from build123d import *

# Parameters (mm, degrees)
EXTRUDE_LID_MAIN_DEPTH = 0.75
EXTRUDE_THIN2_DEPTH    = 0.75
UPPER_17_W             = 5
UPPER_17_H             = 1
UPPER_17_W_2           = 1
UPPER_17_H_2           = 2
LID_ANCHOR_FRONT_DEPTH = 4.5
TAP_LATERAL_LID_D      = 0.75
TAP_FRONT_LID_D        = 0.75
CUT_EXTRUDE1_REACH     = 16.029
HS_HOLDER_LID_DEPTH    = 7.5
M2_5_TAPPED_HOLE2_D    = 2.05


with BuildPart() as part:
    # upper<13> → extrude_lid_main (new body)
    with BuildSketch(Plane(origin=(0, -8, 0), x_dir=(1, 0, 0), z_dir=(0, 1, 0))):
        with BuildLine():
            Line((-6.250353693, -9.5), (6.250353693, -9.5))
            ThreePointArc((6.250353693, -9.5), (7.665029031, -8.913751636), (8.250353267, -7.498693688))
            ThreePointArc((8.250353267, -7.498693688), (8.248836384, -3.124346898), (8.25, 1.25))
            Line((8.25, 1.25), (8.25, 9.2))
            ThreePointArc((8.25, 9.2), (8.162132034, 9.412132034), (7.95, 9.5))
            Line((7.95, 9.5), (0.865, 9.5))
            Line((0.865, 9.5), (0.865, 4.5))
            Line((0.865, 4.5), (-3.935, 4.5))
            Line((-3.935, 4.5), (-3.935, 9.5))
            Line((-3.935, 9.5), (-7.95, 9.5))
            ThreePointArc((-7.95, 9.5), (-8.162132034, 9.412132034), (-8.25, 9.2))
            Line((-8.25, 9.2), (-8.25, 1.25))
            ThreePointArc((-8.25, 1.25), (-8.199296345, -3.106194095), (-8.25, -7.462388189))
            ThreePointArc((-8.25, -7.462388189), (-7.677803101, -8.900852665), (-6.250353693, -9.5))
        make_face()
    extrude(amount=EXTRUDE_LID_MAIN_DEPTH)



with BuildPart() as body_2:
    # upper<16> → Extrude-Thin2 (new body)
    with BuildSketch(Plane(origin=(0, -8, 0), x_dir=(1, 0, 0), z_dir=(0, 1, 0))):
        with BuildLine():
            Line((-8.75, 1.244176388), (-8.75, 9.2))
            ThreePointArc((-8.75, 9.2), (-8.515685425, 9.765685425), (-7.95, 10))
            Line((-7.95, 10), (7.95, 10))
            ThreePointArc((7.95, 10), (8.515685425, 9.765685425), (8.75, 9.2))
            Line((8.75, 9.2), (8.75, 1.249856897))
            ThreePointArc((8.75, 1.249856897), (8.748836381, -3.12425516), (8.75035316, -7.49836711))
            ThreePointArc((8.75035316, -7.49836711), (8.018697866, -9.267189545), (6.250353693, -10))
            Line((6.250353693, -10), (-6.250353693, -10))
            ThreePointArc((-6.250353693, -10), (-8.035078913, -9.250644422), (-8.749889093, -7.451804713))
            ThreePointArc((-8.749889093, -7.451804713), (-8.69929636, -3.103813517), (-8.75, 1.244176388))
        make_face()
        with BuildLine():
            Line((-8.25, 1.25), (-8.25, 9.2))
            ThreePointArc((-8.25, 9.2), (-8.162132034, 9.412132034), (-7.95, 9.5))
            Line((-7.95, 9.5), (7.95, 9.5))
            ThreePointArc((7.95, 9.5), (8.162132034, 9.412132034), (8.25, 9.2))
            Line((8.25, 9.2), (8.25, 1.25))
            ThreePointArc((8.25, 1.25), (8.248836384, -3.124346898), (8.250353267, -7.498693688))
            ThreePointArc((8.250353267, -7.498693688), (7.665029031, -8.913751636), (6.250353693, -9.5))
            Line((6.250353693, -9.5), (-6.250353693, -9.5))
            ThreePointArc((-6.250353693, -9.5), (-7.677803101, -8.900852665), (-8.25, -7.462388189))
            ThreePointArc((-8.25, -7.462388189), (-8.199296345, -3.106194095), (-8.25, 1.25))
        make_face(mode=Mode.SUBTRACT)
    extrude(amount=EXTRUDE_THIN2_DEPTH)


with BuildPart() as part_1:
    add(part.part)

    add(body_2.part)  # lid_anchor_front merges body 2
    # upper<17> → lid_anchor_front (add)
    with BuildSketch(Plane(origin=(0, -8, 0), x_dir=(1, 0, 0), z_dir=(0, 1, 0))):
        with Locations((0, -8.99)):
            Rectangle(UPPER_17_W, UPPER_17_H)
        with Locations((-7.74, 2.25)):
            Rectangle(UPPER_17_W_2, UPPER_17_H_2)
    lid_anchor_front = extrude(amount=-LID_ANCHOR_FRONT_DEPTH)

    # tap_lateral_lid (through all)
    with Locations(Plane.ZY.offset(8.24)):
        with Locations((-2.25, -11)):
            tap_lateral_lid = Hole(TAP_LATERAL_LID_D / 2)

    # Mirror3: lid_anchor_front, tap_lateral_lid across plane
    add(lid_anchor_front.mirror(Plane(origin=(0, 0, 0), x_dir=(0, 0, 1), z_dir=(1, 0, 0))))
    add(tap_lateral_lid.mirror(Plane(origin=(0, 0, 0), x_dir=(0, 0, 1), z_dir=(1, 0, 0))), mode=Mode.SUBTRACT)

    # tap_front_lid (through all)
    with Locations(Plane.XY.offset(9.49)):
        with Locations((0, -9)):
            Hole(TAP_FRONT_LID_D / 2)

    # upper<18> → Cut-Extrude1 (cut, up to next)
    with BuildSketch(Plane(origin=(0, -8, 0), x_dir=(1, 0, 0), z_dir=(0, 1, 0)), mode=Mode.PRIVATE) as cut_extrude1_sk1:
        with BuildLine():
            ThreePointArc((-2.5, 9.5), (-1.767766953, 11.267766953), (0, 12))
            Line((0, 12), (-1.556624327, 12))
            Line((-1.556624327, 12), (-3, 9.5))
            Line((-3, 9.5), (-2.5, 9.5))
        make_face()
    cut_extrude1_tool1 = extrude(cut_extrude1_sk1.sketch, amount=CUT_EXTRUDE1_REACH, mode=Mode.PRIVATE) & part_1.part
    # upper<18> → Cut-Extrude1 (cut, up to next)
    with BuildSketch(Plane(origin=(0, -8, 0), x_dir=(1, 0, 0), z_dir=(0, 1, 0)), mode=Mode.PRIVATE) as cut_extrude1_sk2:
        with BuildLine():
            Line((2.5, 9.5), (3, 9.5))
            Line((3, 9.5), (1.556624327, 12))
            Line((1.556624327, 12), (0, 12))
            ThreePointArc((0, 12), (1.767766953, 11.267766953), (2.5, 9.5))
        make_face()
    cut_extrude1_tool2 = extrude(cut_extrude1_sk2.sketch, amount=CUT_EXTRUDE1_REACH, mode=Mode.PRIVATE) & part_1.part
    # upper<18> → Cut-Extrude1 (cut, up to next)
    with BuildSketch(Plane(origin=(0, -8, 0), x_dir=(1, 0, 0), z_dir=(0, 1, 0)), mode=Mode.PRIVATE) as cut_extrude1_sk3:
        with BuildLine():
            Line((1.25, 9.5), (2.5, 9.5))
            ThreePointArc((2.5, 9.5), (1.767766953, 11.267766953), (0, 12))
            ThreePointArc((0, 12), (-1.767766953, 11.267766953), (-2.5, 9.5))
            Line((-2.5, 9.5), (-1.25, 9.5))
            Line((-1.25, 9.5), (0.865, 9.5))
            Line((0.865, 9.5), (1.25, 9.5))
        make_face()
    cut_extrude1_tool3 = extrude(cut_extrude1_sk3.sketch, amount=CUT_EXTRUDE1_REACH, mode=Mode.PRIVATE) & part_1.part
    # upper<18> → Cut-Extrude1 (cut, up to next)
    with BuildSketch(Plane(origin=(0, -8, 0), x_dir=(1, 0, 0), z_dir=(0, 1, 0)), mode=Mode.PRIVATE) as cut_extrude1_sk4:
        Polygon((1.556624327, 12), (3, 9.5), (3, 12), align=None)
    cut_extrude1_tool4 = extrude(cut_extrude1_sk4.sketch, amount=CUT_EXTRUDE1_REACH, mode=Mode.PRIVATE) & part_1.part
    # upper<18> → Cut-Extrude1 (cut, up to next)
    with BuildSketch(Plane(origin=(0, -8, 0), x_dir=(1, 0, 0), z_dir=(0, 1, 0)), mode=Mode.PRIVATE) as cut_extrude1_sk5:
        Polygon((-3, 9.5), (-1.556624327, 12), (-3.025026025, 12), (-3.025026025, 9.5), align=None)
    cut_extrude1_tool5 = extrude(cut_extrude1_sk5.sketch, amount=CUT_EXTRUDE1_REACH, mode=Mode.PRIVATE) & part_1.part
    add(cut_extrude1_tool1.solids().sort_by_distance((-2.75, -8, -9.539051))[0], mode=Mode.SUBTRACT)
    add(cut_extrude1_tool2.solids().sort_by_distance((2.244493, -8, -10.730474))[0], mode=Mode.SUBTRACT)
    add(cut_extrude1_tool3.solids().sort_by_distance((0, -8, -10.561033))[0], mode=Mode.SUBTRACT)
    add(cut_extrude1_tool4.solids().sort_by_distance((2.518875, -8, -11.166667))[0], mode=Mode.SUBTRACT)
    add(cut_extrude1_tool5.solids().sort_by_distance((-2.535419, -8, -11.152702))[0], mode=Mode.SUBTRACT)

    # upper<25> → hs-holder-lid (add)
    with BuildSketch(Plane(origin=(0, -8, 0), x_dir=(1, 0, 0), z_dir=(0, 1, 0))):
        Polygon((-8.25, 4.5), (-8.25, 3.5), (-2.25, 3.5), (-2.25, 4.5), (-3.935, 4.5), (-4.75, 4.5), align=None)
    hs_holder_lid = extrude(amount=-HS_HOLDER_LID_DEPTH)

    # M2.5 Tapped Hole2 (through all)
    with Locations(Plane(origin=(0, 0, -4.5), x_dir=(-1, 0, 0), z_dir=(0, 0, -1))):
        with Locations((4.25, -10.9)):
            m2_5_tapped_hole2 = Hole(M2_5_TAPPED_HOLE2_D / 2)

    # Mirror6: hs-holder-lid across plane
    add(hs_holder_lid.mirror(Plane(origin=(0, 0, 0), x_dir=(0, 0, 1), z_dir=(1, 0, 0))))

    # Mirror7: M2.5 Tapped Hole2 across plane
    add(m2_5_tapped_hole2.mirror(Plane(origin=(0, 0, 0), x_dir=(0, 0, 1), z_dir=(1, 0, 0))), mode=Mode.SUBTRACT)


solid = part_1.part
Geometry: final body of the model. Coordinates: model frame, mm. A direction names the side the tool comes from. Round coordinates to 2 decimals unless told otherwise and drop trailing zeros. Loops run counter-clockwise (first coordinate to the right, second up) from the corner with the lowest first, then second, coordinate; pieces in that order, holes last.
Q1. Access query for faces 1 (the flat face through (-7.24, -10, -2)), 2 (the flat face through (5, -12, -4.5)), 3 (the flat face through (8, -12.5, -2)), 4 (the flat face through (-5, -12, -3.5)). Directions: +Z, -Z, +X, -X, +Y, -Y. A direction counts if a zero-diameter tool reaches every point of the face in a straight line with its end or side. Return the directions, or none.
Q2. Section C-C on z = -8. Return loops of the section in (x, y) (3 decimals).
Q3. Section B-B on x = 0. Return loops of the section in (y, z) (3 decimals).
Q4. Section A-A on y = -9. Return loops of the section in (x, z) (3 decimals), plus the area to 4 significant figures.
Q5. Section D-D on x = 4.25. Return loops of the section in (y, z) (3 decimals).
Q6. Pin query (flat end, axial travel): P1, Ø4, axis at x = 3.5, y = -13, coming from the -Z side; P2, Ø1.6, axis at x = 4.25, y = -10.9, coming from the -Z side; P3, Ø1.1, axis at x = -1, z = 9, coming from the -Y side; P4, Ø1.1, axis at y = -9.5, z = 9, coming from the -X side. Return the tip coordinate at first contact, or that it passes through.
Q7. Pull-direction query (X, two-part tool) for faces 5 (the flat face through (-2.5, -10, 9)), 6 (the flat face through (8.24, -10, -2)), 7 (the flat face through (2.25, -12, -4)), 8 (the flat face through (-8, -12.5, -2)); classes: released by +X, released by -X, zero draft, split by the parting line, or undercut.
Q8. Material intervals for L1, parallel to Z at x = 7.5, y = -11 (3 decimals); L2, parallel to Y at x = 0, z = 9.15 (3 decimals); L3, parallel to Y at x = -7.95, z = -2.25 (3 decimals), sorted ascending.
Evaluation:
1. face 1: +Z, -Y
1. face 2: -Z, +X, -X, -Y
1. face 3: +Z, +X, -X, -Y
1. face 4: +X, -X, -Y
2. outline: (-8.75, -8) - (-3.935, -8) - (-3.935, -7.25) - (-8.75, -7.25) - close; (0.865, -8) - (8.75, -8) - (8.75, -7.25) - (0.865, -7.25) - close
3. outline: (-12.5, 8.49) - (-9.375, 8.49) - (-9.375, 9.49) - (-12.5, 9.49) - close; (-8.625, 8.49) - (-8, 8.49) - (-8, -4.5) - (-7.25, -4.5) - (-7.25, 10) - (-8, 10) - (-8, 9.49) - (-8.625, 9.49) - close
4. outline: (-8.25, -4.5) - (-2.25, -4.5) - (-2.25, -3.5) - (-8.25, -3.5) - close; (-8.24, -3.25) - (-7.24, -3.25) - (-7.24, -1.25) - (-8.24, -1.25) - close; (-2.5, 8.49) - (-0.375, 8.49) - (-0.375, 9.49) - (-2.5, 9.49) - close; (0.375, 8.49) - (2.5, 8.49) - (2.5, 9.49) - (0.375, 9.49) - close; (2.25, -4.5) - (8.25, -4.5) - (8.25, -3.5) - (2.25, -3.5) - close; (7.24, -3.25) - (8.24, -3.25) - (8.24, -1.25) - (7.24, -1.25) - close
4. area: 20.25 mm2
5. outline: (-15.5, -4.5) - (-11.925, -4.5) - (-11.925, -3.5) - (-15.5, -3.5) - close; (-9.875, -4.5) - (-8, -4.5) - (-8, -10) - (-7.25, -10) - (-7.25, 10) - (-8, 10) - (-8, -3.5) - (-9.875, -3.5) - close
6. P1: stops at z = -4.5
6. P2: passes through
6. P3: stops at y = -12.5
6. P4: stops at x = -2.5
7. face 5: released by -X
7. face 6: released by +X
7. face 7: undercut
7. face 8: zero draft
8. L1: z = -4.5 to -3.5, -3.25 to -2.625, -1.875 to -1.25
8. L2: y = -12.5 to -9.375, -8.625 to -7.25
8. L3: y = -12.5 to -11.375, -10.625 to -7.25
